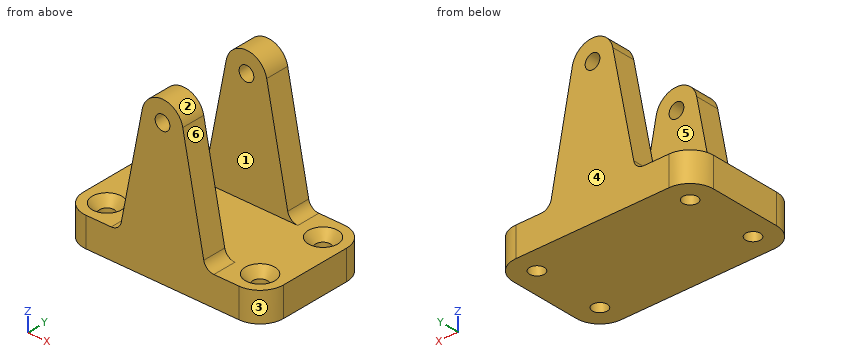
from build123d import *

# Parameters (mm, degrees)
F1_DEPTH = 10
F2_R     = 2.5
F3_DEPTH = 25
F4_R     = 2.5
F5_DEPTH = 8
F6_START = -32
F6_DEPTH = 8


with BuildPart() as f1:
    # F0 (on Top) → F1 (new body)
    with BuildSketch(Plane.XY):
        with BuildLine():
            ThreePointArc((34, 12), (31.6568542495, 17.6568542495), (26, 20))
            Line((26, 20), (-26, 20))
            ThreePointArc((-26, 20), (-31.6568542495, 17.6568542495), (-34, 12))
            Line((-34, 12), (-34, -12))
            ThreePointArc((-34, -12), (-31.6568542495, -17.6568542495), (-26, -20))
            Line((-26, -20), (26, -20))
            ThreePointArc((26, -20), (31.6568542495, -17.6568542495), (34, -12))
            Line((34, -12), (34, 12))
        make_face()
    extrude(amount=-F1_DEPTH)

    # F2 (on face) → F3 (cut)
    with BuildSketch(Plane.XY):
        with Locations((-26, 12)):
            Circle(F2_R)
        with Locations((-26, -12)):
            Circle(F2_R)
        with Locations((26, -12)):
            Circle(F2_R)
        with Locations((26, 12)):
            Circle(F2_R)
    extrude(amount=-F3_DEPTH, mode=Mode.SUBTRACT)

    # F4 (on face) → F5 (join)
    with BuildSketch(Plane.XZ.offset(20)):
        with BuildLine():
            ThreePointArc((6.870243072, 39.3415513897), (6.9674852531, 38.6739059637), (7, 38))
            ThreePointArc((7, 38), (-0.6739059637, 31.0325147469), (-6.870243072, 39.3415513897))
            Line((-6.870243072, 39.3415513897), (-14, 2.8292243052))
            ThreePointArc((-14, 2.8292243052), (-15.2100052393, 0.7983602265), (-17.435121536, 0))
            Line((-17.435121536, 0), (0, 0))
            Line((0, 0), (17.435121536, 0))
            ThreePointArc((17.435121536, 0), (15.2100052393, 0.7983602265), (14, 2.8292243052))
            Line((14, 2.8292243052), (6.870243072, 39.3415513897))
        make_face()
        with BuildLine():
            ThreePointArc((-6.870243072, 39.3415513897), (-0.6739059637, 31.0325147469), (7, 38))
            ThreePointArc((7, 38), (6.9674852531, 38.6739059637), (6.870243072, 39.3415513897))
            ThreePointArc((6.870243072, 39.3415513897), (0, 45), (-6.870243072, 39.3415513897))
        make_face()
        with Locations((0, 38)):
            Circle(F4_R, mode=Mode.SUBTRACT)
    extrude(amount=-F5_DEPTH)

    # F4 (on face) → F6 (join)
    with BuildSketch(Plane.XZ.offset(20).offset(F6_START)):
        with BuildLine():
            ThreePointArc((-6.870243072, 39.3415513897), (-0.6739059637, 31.0325147469), (7, 38))
            ThreePointArc((7, 38), (6.9674852531, 38.6739059637), (6.870243072, 39.3415513897))
            ThreePointArc((6.870243072, 39.3415513897), (0, 45), (-6.870243072, 39.3415513897))
        make_face()
        with Locations((0, 38)):
            Circle(F4_R, mode=Mode.SUBTRACT)
        with BuildLine():
            ThreePointArc((6.870243072, 39.3415513897), (6.9674852531, 38.6739059637), (7, 38))
            ThreePointArc((7, 38), (-0.6739059637, 31.0325147469), (-6.870243072, 39.3415513897))
            Line((-6.870243072, 39.3415513897), (-14, 2.8292243052))
            ThreePointArc((-14, 2.8292243052), (-15.2100052393, 0.7983602265), (-17.435121536, 0))
            Line((-17.435121536, 0), (0, 0))
            Line((0, 0), (17.435121536, 0))
            ThreePointArc((17.435121536, 0), (15.2100052393, 0.7983602265), (14, 2.8292243052))
            Line((14, 2.8292243052), (6.870243072, 39.3415513897))
        make_face()
    extrude(amount=-F6_DEPTH)

    # F8 (on offset) → F9 (revolve, cut)
    with BuildSketch(Plane.XZ.offset(12)):
        Polygon((-21, 0), (-26, 0), (-26, -3), (-23.5, -3), align=None)
    revolve(axis=Axis((-26, -12, -1.5), (0, 0, -1)), mode=Mode.SUBTRACT)

    # F10 (on offset) → F11 (revolve, cut)
    with BuildSketch(Plane.XZ.offset(12)):
        Polygon((31, 0), (26, 0), (26, -3), (28.5, -3), align=None)
    revolve(axis=Axis((26, -12, -1.5), (0, 0, -1)), mode=Mode.SUBTRACT)

    # F13 (on offset) → F14 (revolve, cut)
    with BuildSketch(Plane(origin=(0, 12, 0), x_dir=(-1, 0, 0), z_dir=(0, 1, 0))):
        Polygon((-26, -3), (-26, 0), (-31, 0), (-28.5, -3), align=None)
    revolve(axis=Axis((26, 12, -1.5), (0, 0, -1)), mode=Mode.SUBTRACT)

    # F15 (on offset) → F16 (revolve, cut)
    with BuildSketch(Plane(origin=(0, 12, 0), x_dir=(-1, 0, 0), z_dir=(0, 1, 0))):
        Polygon((31, 0), (26, 0), (26, -3), (28.5, -3), align=None)
    revolve(axis=Axis((-26, 12, -1.5), (0, 0, -1)), mode=Mode.SUBTRACT)


solid = f1.part
Could you check a few things on this model? Use its own coordinates, in mm. Face numbers are marked on the shaded views. A direction names the side the tool comes from. Give positions to 0.01 mm unless a question says otherwise; leave off trailing zeros. Order: outer loops, then holes, each group sorted by start corner. A loop starts at its lowest first (then second) coordinate and runs counter-clockwise, first axis right, second up. Notation, with made-up numbers: (39, 55.5) -> (69, 55.5) arc R21 cw to (69, 74.5) -> close; hole circle Ø1 at (64, -6). An arc over 180 degrees is marked (long way). Return JSON: item names as keys, results as strings.
1. I need wall thicknesses on line 1 (Y direction, x = 26, z = -5); line 2 (X direction, y = 12, z = -5.5); line 3 (Y direction, x = 6, z = 3). Which ranges of each line are inside material? Lowest first, please. Write a range as from..to.
Answer list:
{"line 1": "y = -20..-14.5, -9.5..9.5, 14.5..20", "line 2": "x = -34..-28.5, -23.5..23.5, 28.5..34", "line 3": "y = -20..-12, 12..20"}
2. Imagine slicing it at B-B on z = 38. List the corners of the cut face in (x, y) for me.
Answer list:
{"outline": "(-7.13, -20) -> (-2.5, -20) -> (-2.5, -12) -> (-7.13, -12) -> close; (-7.13, 12) -> (-2.5, 12) -> (-2.5, 20) -> (-7.13, 20) -> close; (2.5, -20) -> (7.13, -20) -> (7.13, -12) -> (2.5, -12) -> close; (2.5, 12) -> (7.13, 12) -> (7.13, 20) -> (2.5, 20) -> close"}
3. Imagine slicing it at D-D on y = -13.5. Give the number of separate pieces and of enclosed holes in the cut face, then the cut area to 3 significant figures.
Answer list:
{"separate pieces": "3", "enclosed holes": "1", "area": "1,460 mm2"}
4. Imagine slicing it at A-A on x = 0. List the corners of the cut face in (y, z) for me, then the cut area to 3 significant figures.
Answer list:
{"outline": "(-20, -10) -> (20, -10) -> (20, 35.5) -> (12, 35.5) -> (12, 0) -> (-12, 0) -> (-12, 35.5) -> (-20, 35.5) -> close; (-20, 40.5) -> (-12, 40.5) -> (-12, 45) -> (-20, 45) -> close; (12, 40.5) -> (20, 40.5) -> (20, 45) -> (12, 45) -> close", "area": "1,040 mm2"}
5. On a 3-axis mill with a long thin cutter (end or side, diameter ignored), from which of +Z, -Z, +X, -X, +Y, -Y can I reach the whole of each face in a straight line? I mean the marked faces 1 and 2. Say none if no direction works.
Answer list:
{"face 1": "+Z, +X, -X", "face 2": "+Z, +Y, -Y"}
6. Thinking about a two-plate mould opening in Y: for the marked faces 3, 4, 5 and 6, which applies, pulls with the +Y half, pulls with the -Y half, needs draft (parallel to the pull), parting line crosses it, or undercut?
Answer list:
{"face 3": "pulls with the -Y half", "face 4": "pulls with the +Y half", "face 5": "undercut", "face 6": "needs draft"}
7. For pin 1 Ø5 at (x, y) = (-18.5, 14) entering from +Z; pin 2 Ø12 at (y, z) = (-10.5, 16.5) entering from -X, each with a flat end and sliding along its axis, tell me the tip position at first contact or that it passes through.
Answer list:
{"pin 1": "stops at z = 0.31", "pin 2": "stops at x = -12.46"}
8. Imagine slicing it at C-C on z = 25.5. List the corners of the cut face in (x, y) for me, then the cut area to 3 significant figures.
Answer list:
{"outline": "(-9.57, -20) -> (9.57, -20) -> (9.57, -12) -> (-9.57, -12) -> close; (-9.57, 12) -> (9.57, 12) -> (9.57, 20) -> (-9.57, 20) -> close", "area": "306 mm2"}
